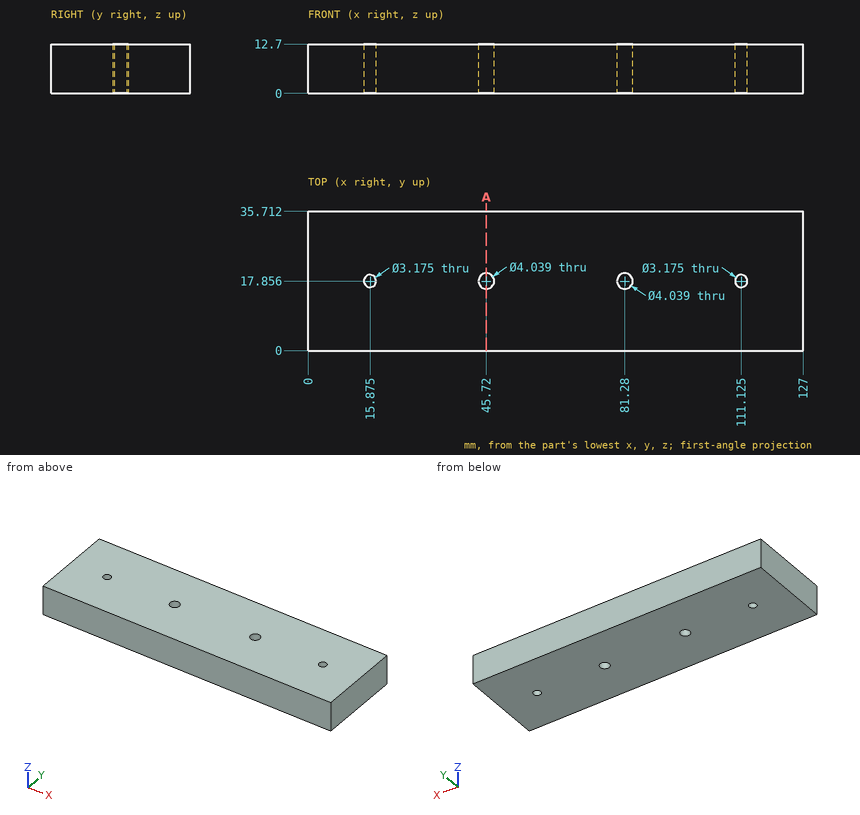
Could you check a few things on this drawing? It's one solid part, dimensions in mm from its lowest x, y, z. Give positions to 0.01 mm unless a question says otherwise; leave off trailing zeros. Order: outer loops, then holes, each group sorted by start corner. A loop starts at its lowest first (then second) coordinate and runs counter-clockwise, first axis right, second up. Notation, with made-up numbers: (-11, -33) - (-4, -33) arc R22 cw to (-4, -22) - close; hole circle Ø7 at (12.25, 69.5). An arc over 180 degrees is marked (long way). Answer as a JSON object with one key per item and string values. Group by question number.
Item 1: For P1, Ø1.9, axis at x = 111.12, y = 17.86, coming from the +Z side, with a flat end and sliding along its axis, tell me the tip position at first contact or that it passes through.
Item 2: Please list where these lines run through material, in increasing order: probe 1 along Y at (x, z) = (16, 11.25); probe 2 along X at (y, z) = (19, 6) (1 decimal); probe 3 along Y at (x, z) = (45.72, 4.25) (1 decimal).
Item 3: If we section it at A-A on x = 45.72: Please give me the cut outline in (y, z) (1 decimal).
Result set:
{
 "1": {"P1": "through"},
 "2": {"probe 1": "0 to 16.27, 19.44 to 35.71", "probe 2": "0 to 14.8, 17 to 44.1, 47.4 to 79.6, 82.9 to 110, 112.2 to 127", "probe 3": "0 to 15.8, 19.9 to 35.7"},
 "3": {"outline": "(0, 0) - (15.8, 0) - (15.8, 12.7) - (0, 12.7) - close; (19.9, 0) - (35.7, 0) - (35.7, 12.7) - (19.9, 12.7) - close"}
}
